```python
from build123d import *

# Parameters (mm, degrees)
EXTRUDE_3_DEPTH     = 21
EXTRUDE_1_DEPTH     = 2.5
SKETCH_9_R          = 1.25
EXTRUDE_2_DEPTH     = 2.5
EXTRUDE_3_2_DEPTH   = 2.5
SKETCH_11_W         = 42
SKETCH_11_H         = 10.406253358
CUT_EXTRUDE_1_DEPTH = 5
FILLET_1_R          = 10
FILLET_2_R          = 2
SKETCH_12_W         = 21.859303669
SKETCH_12_H         = 11.880056341
CUT_EXTRUDE_2_DEPTH = 61
SKETCH_14_R         = 2
CUT_EXTRUDE_3_DEPTH = 10


with BuildPart() as part:
    # 草图7 → Extrude 3 (new, symmetric)
    with BuildSketch(Plane.XY):
        Polygon((51.618317891, 4.889024384), (54.886055332, 4.268404852), (61.410827986, 37.137721863), (10.591755085, 46.789448736), (8.530755399, 35.937702238), (15.711697443, 11.708528829), (19.787318129, 10.93447343), (20.253787963, 13.390569091), (17.675542885, 13.880237947), (11.09997038, 36.066837632), (12.581380912, 43.866883241), (58.467863291, 35.15197032), (52.916660674, 7.187127975), (52.084787725, 7.345120045), align=None)
    extrude(amount=EXTRUDE_3_DEPTH, both=True)

    # 草图8 → 凸台-拉伸1 (add)
    with BuildSketch(Plane.XY.offset(21)):
        Polygon((58.467863291, 35.15197032), (52.916660674, 7.187127975), (52.084787725, 7.345120045), (51.618317891, 4.889024384), (54.886055332, 4.268404852), (61.410827986, 37.137721863), (10.591755085, 46.789448736), (8.530755399, 35.937702238), (15.711697443, 11.708528829), (19.787318129, 10.93447343), (20.253787963, 13.390569091), (17.675542885, 13.880237947), (11.09997038, 36.066837632), (12.581380912, 43.866883241), align=None)
        Polygon((19.787318129, 10.93447343), (51.618317891, 4.889024384), (52.084787725, 7.345120045), (52.916660674, 7.187127975), (58.467863291, 35.15197032), (12.581380912, 43.866883241), (11.09997038, 36.066837632), (17.675542885, 13.880237947), (20.253787963, 13.390569091), align=None)
    extrude(amount=EXTRUDE_1_DEPTH)

    # 草图9 → 凸台-拉伸2 (add)
    with BuildSketch(Plane.XY.offset(-3.5)):
        Polygon((24.397237371, 10.058942279), (26.710927747, 22.241176755), (49.405425881, 17.930962401), (47.091735505, 5.748727924), (54.886055332, 4.268404852), (61.410827986, 37.137721863), (10.591755085, 46.789448736), (8.530755399, 35.937702238), (15.711697443, 11.708528829), align=None)
        with Locations((23.400258978, 16.559120835)):
            Circle(SKETCH_9_R, mode=Mode.SUBTRACT)
        with Locations((50.319067418, 11.446611456)):
            Circle(SKETCH_9_R, mode=Mode.SUBTRACT)
    extrude(amount=EXTRUDE_2_DEPTH)

    # 草图10 → Extrude 3 2 (add)
    with BuildSketch(Plane(origin=(0, 0, -21), x_dir=(-1, 0, 0), z_dir=(0, 0, -1))):
        Polygon((-15.711697443, 11.708528829), (-8.530755399, 35.937702238), (-10.591755085, 46.789448736), (-61.410827986, 37.137721863), (-54.886055332, 4.268404852), align=None)
    extrude(amount=EXTRUDE_3_2_DEPTH)

    # 草图11 → 切除-拉伸1 (cut)
    with BuildSketch(Plane(origin=(17.63296674, 5.225985637, 0), x_dir=(0, 0, 1), z_dir=(-0.9587773323568242, -0.28415845396315786, 0))):
        with Locations((0, 7.59472781)):
            Rectangle(SKETCH_11_W, SKETCH_11_H)
    extrude(amount=-CUT_EXTRUDE_1_DEPTH, mode=Mode.SUBTRACT)

    # 圆角1
    # the kernel refuses this fillet: 10 mm, written as the material it takes off along each edge
    with BuildSketch(Plane(origin=(15.711697443, 11.708528829, -5.758578091), x_dir=(0.9824382642502659, -0.18658793352445072, 0), z_dir=(0, 0, -1)), Plane(origin=(15.711697443, 11.708528829, 38.741421909), x_dir=(0.9824382642502659, -0.18658793352445072, 0), z_dir=(0, 0, -1))) as fillet_1_piece_1:
        with BuildLine():
            CenterArc((FILLET_1_R * 0.609656876359, -FILLET_1_R), FILLET_1_R, 90, 62.737721614)
            Line((-FILLET_1_R * 0.279262123126, -FILLET_1_R * 0.541935580562), (0, 0))
            Line((0, 0), (FILLET_1_R * 0.609656876359, 0))
        make_face()
    extrude(amount=32.982843818, mode=Mode.SUBTRACT)
    with BuildSketch(Plane(origin=(21.237725488, 10.659007254, -17.317640641), x_dir=(0.9824382642502885, -0.18658793352433115, 0), z_dir=(0, 0, 1))) as fillet_1_piece_2:
        with BuildLine():
            CenterArc((6.357442179, 9.493749512), FILLET_1_R, 207.262278386, 44.428504043)
            Line((-2.531747815, 4.913105318), (0, 0))
            Line((0, 0), (3.215990254, 0))
        make_face()
    extrude(amount=30.135281283, mode=Mode.SUBTRACT)
    with BuildSketch(Plane(origin=(8.530755399, 35.937702238, 29.562520674), x_dir=(0.18658793352445296, 0.9824382642502654, 0), z_dir=(0, 0, -1))) as fillet_1_piece_3:
        with BuildLine():
            CenterArc((FILLET_1_R * 0.242500826961, FILLET_1_R), FILLET_1_R, 242.737721614, 27.262278386)
            Line((-FILLET_1_R * 0.215563592477, FILLET_1_R * 0.111081000515), (0, 0))
            Line((0, 0), (FILLET_1_R * 0.242500826961, 0))
        make_face()
    extrude(amount=59.125041348, mode=Mode.SUBTRACT)

    # 圆角2
    fillet_2_edges = [part.edges().sort_by_distance(p)[0] for p in [
        (36.001291535, 41.963585299, -23.5),
        (58.148441659, 20.703063357, -23.5),
        (38.293627604, 7.419693757, -23.5),
        (11.599573944, 25.583220021, 23.5),
        (11.599573944, 25.583220021, -23.5),
        (9.787493883, 42.554785944, -23.5),
        (16.859888508, 12.978250443, -23.5),
        (8.820223079, 35.952251632, -23.5),
        (38.293627604, 7.419693757, 23.5),
        (16.859888508, 12.978250443, 23.5),
        (8.820223079, 35.952251632, 23.5),
        (54.886055332, 4.268404852, 0),
        (58.148441659, 20.703063357, 23.5),
        (36.001291535, 41.963585299, 23.5),
        (9.787493883, 42.554785944, 23.5),
    ]]
    fillet(fillet_2_edges, radius=FILLET_2_R)

    # 草图12 → 切除-拉伸2 (cut)
    with BuildSketch(Plane(origin=(8.479309234, 44.645962299, 0), x_dir=(0.9824382642502656, -0.18658793352445194, 0), z_dir=(-0.18658793352445194, -0.9824382642502656, 0))):
        with Locations((32.525954901, 11.00026169)):
            Rectangle(SKETCH_12_W, SKETCH_12_H)
    extrude(amount=-CUT_EXTRUDE_2_DEPTH, mode=Mode.SUBTRACT)

    # 草图14 → 切除-拉伸3 (cut)
    with BuildSketch(Plane(origin=(0, 0, -23.5), x_dir=(-1, 0, 0), z_dir=(0, 0, -1))):
        with Locations((-50.319067418, 11.446611456)):
            Circle(SKETCH_14_R)
        with Locations((-23.400258978, 16.559120835)):
            Circle(SKETCH_14_R)
    extrude(amount=-CUT_EXTRUDE_3_DEPTH, mode=Mode.SUBTRACT)


solid = part.part
```
Geometry: final body of the model. Coordinates: model frame, mm. A direction names the side the tool comes from. Round coordinates to 2 decimals unless told otherwise and drop trailing zeros. Write each loop counter-clockwise with the first axis right and the second up, starting at its lowest first coordinate (ties: lowest second). Pieces come first, ordered by that corner, then holes. Notation, with made-up numbers: M -5.75,-38 L 8.25,-38 A23 cw 8.25,-16 Z; hole C 11,45 d6. An arc over 180 degrees is marked long. Answer in a Markdown table with one row per item. Add a question column.
(1) Reachability of faces 1 (the face through (51.79, 12.8, -22.27)), 2 (the face through (34, 29, -3.5)), 3 (the face through (21.419, 12.587, -2.268)) from +Z, -Z, +X, -X, +Y, -Y: full face, straight path, thin tool, end or side. Return the list, or none.
(2) Draft query along Z for faces 4 (the face through (58.385, 21.892, 0.301)), 5 (the face through (12.18, 25.63, 22.9)), 6 (the face through (51.4, 37.75, 10.92)). Return one class per face: pulls with the +Z half, pulls with the -Z half, needs draft (parallel to the pull), parting line crosses it, or undercut.
(3) Cut plane A-A, the plane z = 3.5. Return the cut outline in (x, y).
(4) Cut plane C-C, the plane z = 14. Return the cut outline in (x, y), then the cut area to 3 significant figures.
(5) Ray query, L1, parallel to Z at x = 19.5, y = 31; L2, parallel to Z at x = 28, y = 19; L3, parallel to Z at x = 44, y = 40. Return the intervals inside material, ascending.
(6) Cut plane B-B, the plane z = -2.5. Return the cut outline in (x, y).
(7) Contact query for flat-ended pins moving along their axis: pin 1 (6 mm diameter, centred on y = 20, z = 15.5, fed in from -X); pin 2 (8 mm diameter, centred on x = 54.5, z = 13.5, fed in from +Y); pin 3 (1 mm diameter, centred on y = 39, z = 10.5, fed in from -X). Output: stop coordinate, or through.
(8) Cut plane D-D, the plane y = 26. Give the number of separate pieces and of enclosed holes in the cut face, then the cut area to 3 significant figures.
Established:
| question | item | result |
|---|---|---|
| 1 | face 1 | -Z |
| 1 | face 2 | none |
| 1 | face 3 | -X, -Y |
| 2 | face 4 | needs draft |
| 2 | face 5 | pulls with the +Z half |
| 2 | face 6 | undercut |
| 3 | outline | M 8.98,38.32 A10 ccw 9.22,33.61 L 14,17.5 L 16.39,18.21 L 11.1,36.07 L 12.58,43.87 L 58.47,35.15 L 52.92,7.19 L 52.08,7.35 L 51.62,4.89 L 52.94,4.64 A2 ccw 55.27,6.21 L 61.41,37.14 L 10.59,46.79 Z |
| 4 | outline | M 8.98,38.32 A10 ccw 9.22,33.61 L 13.98,17.55 A10 ccw 14,17.5 L 16.39,18.21 L 11.1,36.07 L 12.58,43.87 L 29.7,40.62 L 30.16,43.07 L 10.59,46.79 Z; M 51.17,36.54 L 58.47,35.15 L 52.92,7.19 L 52.08,7.35 L 51.62,4.89 L 52.94,4.64 A2 ccw 55.27,6.21 L 61.41,37.14 L 51.64,38.99 Z |
| 4 | area | 221 mm² |
| 5 | L1 | -23.5 to -21, -3.5 to -1, 21 to 23.5 |
| 5 | L2 | -23.5 to -21, 21 to 23.5 |
| 5 | L3 | -22.75 to 5.06, 16.94 to 22.75 |
| 6 | outline | M 8.98,38.32 A10 ccw 9.22,33.61 L 14,17.5 L 18.79,18.92 L 19.67,15.96 A10 ccw 24.4,10.06 L 26.71,22.24 L 49.41,17.93 L 47.09,5.75 L 52.94,4.64 A2 ccw 55.27,6.21 L 61.41,37.14 L 10.59,46.79 Z; hole C 23.4,16.56 d2.5; hole C 50.32,11.45 d2.5 |
| 7 | pin 1 | x = 12.37 |
| 7 | pin 2 | y = 38.99 |
| 7 | pin 3 | x = 9.02 |
| 8 | separate pieces | 1 |
| 8 | enclosed holes | 2 |
| 8 | area | 558 mm² |
